The figure shows three views and two pictorial views of one solid part (mm, origin at its lowest corner). Answer the questions. A direction names the side the tool comes from. Round coordinates to 2 decimals unless told otherwise and drop trailing zeros. Write each loop counter-clockwise with the first axis right and the second up, starting at its lowest first coordinate (ties: lowest second). Pieces come first, ordered by that corner, then holes. Notation, with made-up numbers: M 4,89.25 L 17,89.25 A20 ccw 17,94.25 Z; hole C 56,31 d5. An arc over 180 degrees is marked long. Answer in a Markdown table with one row per item.
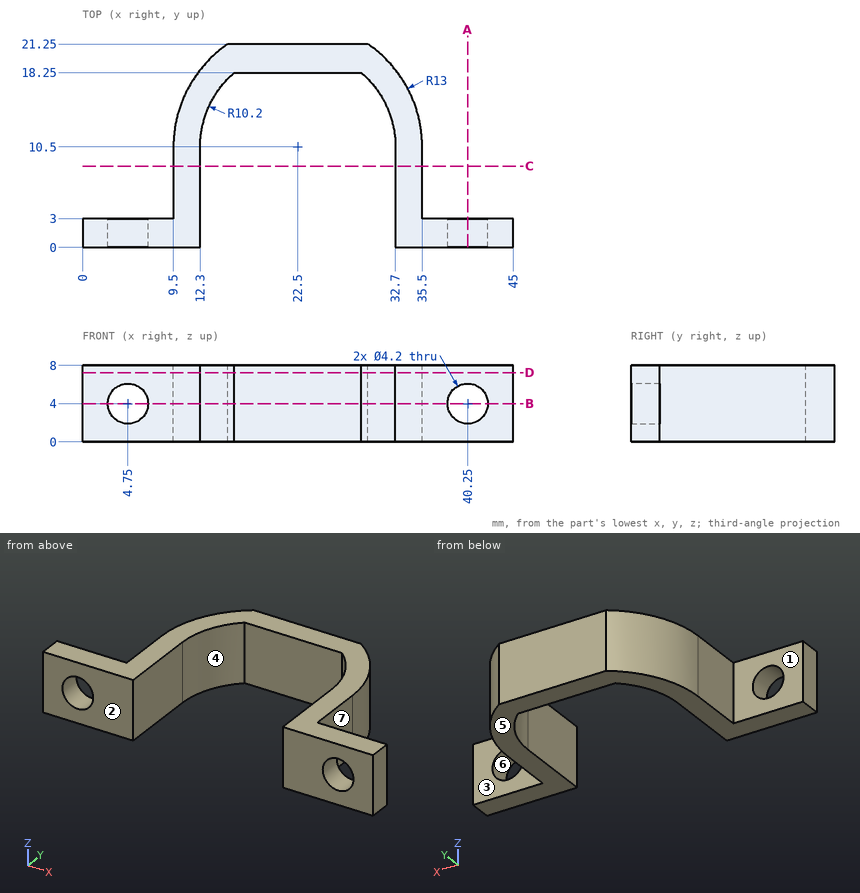
1. Consider line 1 along X through (y, z) = (0.9, 4); line 2 along X through (y, z) = (7.5, 6.25); line 3 along Y through (x, z) = (41, 1.5). Determine where each line is inside the solid, lowest interval first. Write a range as from..to.
Calculated:
| item | result |
|---|---|
| line 1 | x = 0..2.65, 6.85..12.3, 32.7..38.15, 42.35..45 |
| line 2 | x = 9.5..12.3, 32.7..35.5 |
| line 3 | y = 0..3 |
2. The part is cut by section D-D (z = 7.25). Determine the outline of the cut face in (x, y), plus the area to 3 significant figures.
Calculated:
| item | result |
|---|---|
| outline | M 0,0 L 12.3,0 L 12.3,10.5 A10.2 cw 15.87,18.25 L 29.13,18.25 A10.2 cw 32.7,10.5 L 32.7,0 L 45,0 L 45,3 L 35.5,3 L 35.5,10.5 A13 ccw 29.81,21.25 L 15.19,21.25 A13 ccw 9.5,10.5 L 9.5,3 L 0,3 Z |
| area | 218 mm² |
3. The part is cut by section C-C (y = 8.5). Determine the outline of the cut face in (x, z).
Calculated:
| item | result |
|---|---|
| outline | M 9.5,0 L 12.3,0 L 12.3,8 L 9.5,8 Z; M 32.7,0 L 35.5,0 L 35.5,8 L 32.7,8 Z |
4. Given pin 1 (1 mm diameter, centred on y = 8, z = 7, fed in from +X); pin 2 (1 mm diameter, centred on y = 17.5, z = 3, fed in from -X); pin 3 (1 mm diameter, centred on y = 17, z = 6, fed in from -X), each flat-ended and moving along its own axis, determine where each tip first touches the part or whether it passes through.
Calculated:
| item | result |
|---|---|
| pin 1 | stops at x = 35.5 |
| pin 2 | stops at x = 11.24 |
| pin 3 | stops at x = 10.97 |
5. The part is cut by section A-A (x = 40.25). Determine the outline of the cut face in (y, z).
Calculated:
| item | result |
|---|---|
| outline | M 0,0 L 3,0 L 3,1.9 L 0,1.9 Z; M 0,6.1 L 3,6.1 L 3,8 L 0,8 Z |
6. Determine the mould class of the marked faces 5, 6 and 7 for opening direction Z: released by +Z, released by -Z, zero draft, split by the parting line, or undercut.
Calculated:
| item | result |
|---|---|
| face 5 | released by -Z |
| face 6 | undercut |
| face 7 | zero draft |
7. A tool of negligible diameter and unlimited length cuts with its end or side. For the marked faces 1, 2, 3 and 4, from which of +Z, -Z, +X, -X, +Y, -Y can it reach the whole face along a straight path? Write none if from no direction.
Calculated:
| item | result |
|---|---|
| face 1 | +Z, -Z, -X, +Y |
| face 2 | +Z, -Z, +X, -X, -Y |
| face 3 | +Z, -Z, +X, +Y |
| face 4 | +Z, -Z, -Y |
8. The part is cut by section B-B (z = 4). Determine the outline of the cut face in (x, y).
Calculated:
| item | result |
|---|---|
| outline | M 0,0 L 2.65,0 L 2.65,3 L 0,3 Z; M 6.85,0 L 12.3,0 L 12.3,10.5 A10.2 cw 15.87,18.25 L 29.13,18.25 A10.2 cw 32.7,10.5 L 32.7,0 L 38.15,0 L 38.15,3 L 35.5,3 L 35.5,10.5 A13 ccw 29.81,21.25 L 15.19,21.25 A13 ccw 9.5,10.5 L 9.5,3 L 6.85,3 Z; M 42.35,0 L 45,0 L 45,3 L 42.35,3 Z |
